Can you work these out from the model? Positions are in its coordinate system, mm. A direction names the side the tool comes from. Round coordinates to 2 decimals unless told otherwise and drop trailing zeros. Order: outer loops, then holes, each group sorted by start corner. A loop starts at its lowest first (then second) coordinate and runs counter-clockwise, first axis right, second up.
from build123d import *

# Parameters (mm, degrees)
F0_W      = 43.5
F0_H      = 43.5
F0_R      = 1.5
F1_DEPTH  = 1.5
F2_W      = 23
F2_H      = 16
F3_DEPTH  = 24.5
F4_W      = 8
F4_H      = 2.5
F5_DEPTH  = 2.3
F6_W      = 5.75
F6_H      = 5.75
F7_DEPTH  = 2
F8_R      = 4
F9_DEPTH  = 11
F10_W     = 7.5
F10_H     = 10
F10_W_2   = 15
F10_H_2   = 7.5
F11_DEPTH = 10
F12_W     = 14
F12_H     = 5
F13_DEPTH = 8.5
F14_W     = 2.5
F14_H     = 2.3
F15_DEPTH = 0.2
F16_W     = 2.5
F16_H     = 2.3
F17_DEPTH = 0.2


with BuildPart() as f1:
    # F0 (on Top) → F1 (new body)
    with BuildSketch(Plane.XY):
        Rectangle(F0_W, F0_H)
        with Locations((-18.75, -18.75)):
            Circle(F0_R, mode=Mode.SUBTRACT)
        with Locations((18.75, -18.75)):
            Circle(F0_R, mode=Mode.SUBTRACT)
        with Locations((-18.75, 18.75)):
            Circle(F0_R, mode=Mode.SUBTRACT)
        with Locations((18.75, 18.75)):
            Circle(F0_R, mode=Mode.SUBTRACT)
    extrude(amount=F1_DEPTH)

    # F2 (on face) → F3 (join)
    with BuildSketch(Plane.XY.offset(1.5)):
        with Locations((0.25, 13.75)):
            Rectangle(F2_W, F2_H)
    extrude(amount=F3_DEPTH)

    # F4 (on face) → F5 (join)
    with BuildSketch(Plane.XY.offset(1.5)):
        with Locations((-17.75, 13.25)):
            Rectangle(F4_W, F4_H)
        with Locations((-17.75, 9.5)):
            Rectangle(F4_W, F4_H)
        with Locations((-17.75, 5)):
            Rectangle(F4_W, F4_H)
        with Locations((17.75, 13.25)):
            Rectangle(F4_W, F4_H)
        with Locations((17.75, 9.5)):
            Rectangle(F4_W, F4_H)
        with Locations((17.75, 5)):
            Rectangle(F4_W, F4_H)
        with Locations((17.75, 1.25)):
            Rectangle(F4_W, F4_H)
        with Locations((-17.75, 1.25)):
            Rectangle(F4_W, F4_H)
    extrude(amount=F5_DEPTH)

    # F6 (on face) → F7 (join)
    with BuildSketch(Plane.XY.offset(1.5)):
        with Locations((6.375, -2.875)):
            Rectangle(F6_W, F6_H)
    extrude(amount=F7_DEPTH)

    # F8 (on face) → F9 (join)
    with BuildSketch(Plane.XY.offset(1.5)):
        with Locations((-6.25, -3.75)):
            Circle(F8_R)
        with Locations((6.75, -10.55)):
            Circle(F8_R)
    extrude(amount=F9_DEPTH)

    # F10 (on face) → F11 (join)
    with BuildSketch(Plane.XY.offset(1.5)):
        with Locations((16.7, -6.75)):
            Rectangle(F10_W, F10_H)
        with Locations((-16.7, -6.75)):
            Rectangle(F10_W, F10_H)
        with Locations((-7.75, -16.7)):
            Rectangle(F10_W_2, F10_H_2)
    extrude(amount=F11_DEPTH)

    # F12 (on face) → F13 (join)
    with BuildSketch(Plane.XY.offset(1.5)):
        with Locations((8.75, -17.75)):
            Rectangle(F12_W, F12_H)
    extrude(amount=F13_DEPTH)

    # F14 (on face) → F15 (cut)
    with BuildSketch(Plane.YZ.offset(21.75)):
        with Locations((1.25, 2.65)):
            Rectangle(F14_W, F14_H)
        with Locations((5, 2.65)):
            Rectangle(F14_W, F14_H)
        with Locations((9.5, 2.65)):
            Rectangle(F14_W, F14_H)
        with Locations((13.25, 2.65)):
            Rectangle(F14_W, F14_H)
    extrude(amount=-F15_DEPTH, mode=Mode.SUBTRACT)

    # F16 (on face) → F17 (cut)
    with BuildSketch(Plane(origin=(-21.75, 0, 0), x_dir=(0, -1, 0), z_dir=(-1, 0, 0))):
        with Locations((-13.25, 2.65)):
            Rectangle(F16_W, F16_H)
        with Locations((-9.5, 2.65)):
            Rectangle(F16_W, F16_H)
        with Locations((-5, 2.65)):
            Rectangle(F16_W, F16_H)
        with Locations((-1.25, 2.65)):
            Rectangle(F16_W, F16_H)
    extrude(amount=-F17_DEPTH, mode=Mode.SUBTRACT)


solid = f1.part
(1) On a 3-axis mill with a long thin cutter (end or side, diameter ignored), from which of +Z, -Z, +X, -X, +Y, -Y can I reach the whole of each face in a straight line? I mean faces 5 (the face through (-7.117, -7.655, 6.923)), 6 (the face through (17, -7, 11.5)), 7 (the face through (-18, 10.75, 3)). Say none if no direction works.
(2) I'm going to push flat-ended pins straight in: pin 1 Ø5 at (y, z) = (-6.5, 8) entering from +X; pin 2 Ø7 at (x, z) = (4, 8.5) entering from -Y; pin 3 Ø13 at (y, z) = (11, 9.5) entering from -X. Where does each tip first touch, or does it pass through?
(3) If we mould it in two halves opening along X, with no side actions, what happens to faces 1 (the face through (-21.55, 1, 3)), 2 (the face through (21.55, 13, 3)), 3 (the face through (0, 0, 0)), 4 (the face through (-13.75, 13, 3))? For each: pulls with the +X half, pulls with the -X half, needs draft (parallel to the pull), parting line crosses it, or undercut.
(4) Please list where these lines run through material, in increasing order: probe 1 along Y at (x, z) = (-18.75, 0.85); probe 2 along Y at (x, z) = (8, 7.25); probe 3 along Y at (x, z) = (-3.5, 23.5).
(5) I want a section at B-B, the plane x = 18.75. Give the number of separate pieces and of enclosed holes in the cut face, plus the area to 3 significant figures.
(6) I want a section at C-C, the plane z = 8. List the corners of the cut face in (x, y) for me.
(7) I want a section at D-D, the plane y = -10.55. List the corners of the cut face in (x, z) for me, plus the area to 3 significant figures.
(8) I want a section at A-A, the plane y = -18.75. List the corners of the cut face in (x, z) for me, plus the area to 3 significant figures.
Ans:
1. face 5: +Z
1. face 6: +Z, +X, +Y, -Y
1. face 7: +Z, -X
2. pin 1: stops at x = 20.45
2. pin 2: stops at y = -20.25
2. pin 3: stops at x = -21.55
3. face 1: pulls with the -X half
3. face 2: pulls with the +X half
3. face 3: needs draft
3. face 4: undercut
4. probe 1: y = -21.75 to -20.25, -17.25 to 17.25, 20.25 to 21.75
4. probe 2: y = -20.25 to -15.25, -14.35 to -6.75, 5.75 to 21.75
4. probe 3: y = 5.75 to 21.75
5. separate pieces: 3
5. enclosed holes: 0
5. area: 179 mm2
6. outline: (-20.45, -11.75) - (-12.95, -11.75) - (-12.95, -1.75) - (-20.45, -1.75) - close; (-15.25, -20.45) - (-0.25, -20.45) - (-0.25, -12.95) - (-15.25, -12.95) - close; (-11.25, 5.75) - (11.75, 5.75) - (11.75, 21.75) - (-11.25, 21.75) - close; circle Ø8 at (-6.25, -3.75); (1.75, -20.25) - (15.75, -20.25) - (15.75, -15.25) - (1.75, -15.25) - close; circle Ø8 at (6.75, -10.55); (12.95, -11.75) - (20.45, -11.75) - (20.45, -1.75) - (12.95, -1.75) - close
7. outline: (-21.75, 0) - (21.75, 0) - (21.75, 1.5) - (20.45, 1.5) - (20.45, 11.5) - (12.95, 11.5) - (12.95, 1.5) - (10.75, 1.5) - (10.75, 12.5) - (2.75, 12.5) - (2.75, 1.5) - (-12.95, 1.5) - (-12.95, 11.5) - (-20.45, 11.5) - (-20.45, 1.5) - (-21.75, 1.5) - close
7. area: 303 mm2
8. outline: (-21.75, 0) - (-20.25, 0) - (-20.25, 1.5) - (-21.75, 1.5) - close; (-17.25, 0) - (17.25, 0) - (17.25, 1.5) - (15.75, 1.5) - (15.75, 10) - (1.75, 10) - (1.75, 1.5) - (-0.25, 1.5) - (-0.25, 11.5) - (-15.25, 11.5) - (-15.25, 1.5) - (-17.25, 1.5) - close; (20.25, 0) - (21.75, 0) - (21.75, 1.5) - (20.25, 1.5) - close
8. area: 325 mm2
